from build123d import *

# Parameters (mm, degrees)
F0_W      = 60
F0_H      = 30
F1_DEPTH  = 150
F2_T      = -2
F4_D      = 3
F3_R      = 11
F5_DEPTH  = 30.001
F6_D      = 3
F7_D      = 3
F8_W      = 52
F8_H      = 31
F8_R      = 1.5
F8_W_2    = 60
F8_H_2    = 85.5
F8_R_2    = 11
F8_W_3    = 15
F8_H_3    = 25.5
F8_W_4    = 22.5
F9_DEPTH  = 25
F10_DEPTH = 30.001
F11_F1_R  = 4
F11_F2_R  = 4
F11_F3_R  = 4
F11_F4_R  = 4
F11_F5_R  = 4
F11_F6_R  = 4
F11_F7_R  = 4
F11_F8_R  = 4
F11_F9_R  = 4
F11_F10_R = 4
F11_F11_R = 4


with BuildPart() as f1:
    # F0 (on Top) → F1 (new body)
    with BuildSketch(Plane.XY):
        Rectangle(F0_W, F0_H)
    extrude(amount=F1_DEPTH)

    # F2
    f2_openings = [f1.faces().sort_by_distance(p)[0] for p in [
        (0, 0, 150),
        (0, 0, 0),
    ]]
    offset(amount=F2_T, openings=f2_openings)

    # F4 (through all)
    with Locations(Plane(origin=(0, 15, 0), x_dir=(-1, 0, 0), z_dir=(0, 1, 0))):
        with Locations((-12.5, 117.5), (12.5, 117.5), (-12.5, 92.5), (12.5, 92.5)):
            Hole(F4_D / 2)

    # F3 (on face) → F5 (cut, through all)
    with BuildSketch(Plane(origin=(0, 15, 0), x_dir=(-1, 0, 0), z_dir=(0, 1, 0))):
        with Locations((0, 55)):
            Circle(F3_R)
    extrude(amount=-F5_DEPTH, mode=Mode.SUBTRACT)

    # F6 (through all)
    with Locations(Plane(origin=(0, 15, 0), x_dir=(-1, 0, 0), z_dir=(0, 1, 0))):
        with Locations((-15.5, 70.5), (15.5, 70.5), (-15.5, 39.5), (15.5, 39.5)):
            Hole(F6_D / 2)

    # F7 (through all)
    with Locations(Plane(origin=(0, 15, 0), x_dir=(-1, 0, 0), z_dir=(0, 1, 0))):
        with Locations((-2, 141), (1, 134)):
            Hole(F7_D / 2)

    # F8 (on face) → F9 (cut)
    with BuildSketch(Plane.XZ.offset(15)):
        with Locations((0, 105)):
            Rectangle(F8_W, F8_H)
        with Locations((-12.5, 92.5)):
            Circle(F8_R, mode=Mode.SUBTRACT)
        with Locations((-12.5, 117.5)):
            Circle(F8_R, mode=Mode.SUBTRACT)
        with Locations((12.5, 92.5)):
            Circle(F8_R, mode=Mode.SUBTRACT)
        with Locations((12.5, 117.5)):
            Circle(F8_R, mode=Mode.SUBTRACT)
        with Locations((0, 42.75)):
            Rectangle(F8_W_2, F8_H_2)
        with Locations((-15.5, 39.5)):
            Circle(F8_R, mode=Mode.SUBTRACT)
        with Locations((-15.5, 70.5)):
            Circle(F8_R, mode=Mode.SUBTRACT)
        with Locations((0, 55)):
            Circle(F8_R_2, mode=Mode.SUBTRACT)
        with Locations((15.5, 39.5)):
            Circle(F8_R, mode=Mode.SUBTRACT)
        with Locations((15.5, 70.5)):
            Circle(F8_R, mode=Mode.SUBTRACT)
        with Locations((0, 137.25)):
            Rectangle(F8_W_3, F8_H_3)
        with Locations((-1, 134)):
            Circle(F8_R, mode=Mode.SUBTRACT)
        with Locations((2, 141)):
            Circle(F8_R, mode=Mode.SUBTRACT)
        with Locations((18.75, 137.25)):
            Rectangle(F8_W_4, F8_H_3)
        with Locations((-18.75, 137.25)):
            Rectangle(F8_W_4, F8_H_3)
    extrude(amount=-F9_DEPTH, mode=Mode.SUBTRACT)

    # F8 (on face) → F10 (cut, through all)
    with BuildSketch(Plane.XZ.offset(15)):
        with Locations((-18.75, 137.25)):
            Rectangle(F8_W_4, F8_H_3)
        with Locations((18.75, 137.25)):
            Rectangle(F8_W_4, F8_H_3)
    extrude(amount=-F10_DEPTH, mode=Mode.SUBTRACT)

    # F11: fillet of radius 4 on 12 edges, made by hand

    # F11_f1
    f11_f1_edges = [f1.edges().sort_by_distance(p)[0] for p in [
        (29, 10, 0),
    ]]
    fillet(f11_f1_edges, radius=F11_F1_R)

    # F11_f2
    f11_f2_edges = [f1.edges().sort_by_distance(p)[0] for p in [
        (29, 10, 85.5),
    ]]
    fillet(f11_f2_edges, radius=F11_F2_R)

    # F11_f3
    f11_f3_edges = [f1.edges().sort_by_distance(p)[0] for p in [
        (7.5, 14, 124.5),
    ]]
    fillet(f11_f3_edges, radius=F11_F3_R)

    # F11_f4
    f11_f4_edges = [f1.edges().sort_by_distance(p)[0] for p in [
        (7.5, 14, 150),
    ]]
    fillet(f11_f4_edges, radius=F11_F4_R)

    # F11_f5
    f11_f5_edges = [f1.edges().sort_by_distance(p)[0] for p in [
        (-7.5, 14, 150),
    ]]
    fillet(f11_f5_edges, radius=F11_F5_R)

    # F11_f6
    f11_f6_edges = [f1.edges().sort_by_distance(p)[0] for p in [
        (-7.5, 14, 124.5),
    ]]
    fillet(f11_f6_edges, radius=F11_F6_R)

    # F11_f7
    f11_f7_edges = [f1.edges().sort_by_distance(p)[0] for p in [
        (-29, 10, 85.5),
    ]]
    fillet(f11_f7_edges, radius=F11_F7_R)

    # F11_f8
    f11_f8_edges = [f1.edges().sort_by_distance(p)[0] for p in [
        (26, -14, 89.5),
    ]]
    fillet(f11_f8_edges, radius=F11_F8_R)

    # F11_f9
    f11_f9_edges = [f1.edges().sort_by_distance(p)[0] for p in [
        (-26, -14, 89.5),
    ]]
    fillet(f11_f9_edges, radius=F11_F9_R)

    # F11_f10
    f11_f10_edges = [f1.edges().sort_by_distance(p)[0] for p in [
        (-26, -14, 120.5),
    ]]
    fillet(f11_f10_edges, radius=F11_F10_R)

    # F11_f11
    f11_f11_edges = [f1.edges().sort_by_distance(p)[0] for p in [
        (26, -14, 120.5),
    ]]
    fillet(f11_f11_edges, radius=F11_F11_R)


solid = f1.part
Work out the finished part from the listing and answer in its coordinate system (mm). A direction names the side the tool comes from. Give positions to 0.01 mm unless a question says otherwise; leave off trailing zeros. Loops run counter-clockwise (first coordinate to the right, second up) from the corner with the lowest first, then second, coordinate; pieces in that order, holes last. Notation, with made-up numbers: (1.25, 36.25) - (46.25, 36.25) arc R25 ccw to (46.25, 71.25) - close; hole circle Ø9 at (35, 77.25). An arc over 180 degrees is marked (long way). Answer in a Markdown table with one row per item. Add a question column.
Q1. A tool of negligible diameter and unlimited length cuts with its end or side. For faces 4 (the flat face through (28, 3, 89)), 5 (the cylindrical face through (8.703, 14.014, 125.641)), 6 (the cylindrical face through (24.797, -13.986, 119.359)), from which of +Z, -Z, +X, -X, +Y, -Y can it reach the whole face along a straight path? Write none if from no direction.
Q2. Each of these flat-tipped pins is pushed along its axis until it touches: P1, Ø4, axis at x = -1, z = 134, coming from the -Y side; P2, Ø1.6, axis at x = -0.5, y = -13.5, coming from the -Z side; P3, Ø4, axis at x = 18.5, z = 127.5, coming from the -Y side; P4, Ø1, axis at x = -29, z = 32, coming from the -Y side. Where does it stop, or does it pass through?
Q3. The part is cut by section A-A (z = 134). Determine the outline of the cut face in (x, y), and give its area (3 significant figures).
Q4. Determine the mould class of faces 1 (the flat face through (30, 3, 89)), 2 (the flat face through (0, -14, 85.5)), 3 (the cylindrical face through (15.305, 13.986, 71.987)) for opening direction X: released by +X, released by -X, zero draft, split by the parting line, or undercut.
Q5. Consider line 1 along Z through (x, y) = (-12.5, 13.9); line 2 along X through (y, z) = (14.55, 117.5); line 3 along X through (y, z) = (10.75, 115.5). Determine where each line is inside the solid, lowest interval first.
Q6. The part is cut by section C-C (x = 20). Determine the outline of the cut face in (y, z), and give its area (3 significant figures).
Q7. The part is cut by section B-B (y = 0). Determine the outline of the cut face in (x, z).
Q8. The part is cut by section D-D (z = 35). Determine the outline of the cut face in (x, y).
Solution:
| question | item | result |
|---|---|---|
| 1 | face 4 | +Z, -Z |
| 1 | face 5 | +Z, +X, +Y, -Y |
| 1 | face 6 | -Y |
| 2 | P1 | stops at y = 13 |
| 2 | P2 | stops at z = 85.5 |
| 2 | P3 | passes through |
| 2 | P4 | stops at y = 10 |
| 3 | outline | (-7.5, 13) - (-2.5, 13) - (-2.5, 15) - (-7.5, 15) - close; (0.5, 13) - (7.5, 13) - (7.5, 15) - (0.5, 15) - close |
| 3 | area | 24.0 mm² |
| 4 | face 1 | released by +X |
| 4 | face 2 | zero draft |
| 4 | face 3 | undercut |
| 5 | line 1 | z = 0 to 91, 94 to 116, 119 to 124.5 |
| 5 | line 2 | x = -30 to -14, -11 to 11, 14 to 30 |
| 5 | line 3 | x = -30 to -28, 28 to 30 |
| 6 | outline | (-15, 85.5) - (-13, 85.5) - (-13, 89.5) - (-15, 89.5) - close; (-15, 120.5) - (-13, 120.5) - (-13, 124.5) - (-15, 124.5) - close; (13, 0.13) arc R4 ccw to (14, 0) - (15, 0) - (15, 124.5) - (13, 124.5) - close |
| 6 | area | 265 mm² |
| 7 | outline | (-30, 85.5) - (-28, 85.5) - (-28, 124.5) - (-30, 124.5) - close; (28, 85.5) - (30, 85.5) - (30, 124.5) - (28, 124.5) - close |
| 8 | outline | (-30, 10) - (-28, 10) - (-28, 13) - (28, 13) - (28, 10) - (30, 10) - (30, 15) - (-30, 15) - close |
